Verification items for this drawing (mm, ordinates from the low corner). Round coordinates to 2 decimals unless told otherwise and drop trailing zeros. Loops run counter-clockwise (first coordinate to the right, second up) from the corner with the lowest first, then second, coordinate; pieces in that order, holes last. Notation, with made-up numbers: (28, 67) -> (65, 67) arc R24 cw to (65, 84) -> close; hole circle Ø1 at (77, 22). An arc over 180 degrees is marked (long way). Use a Markdown table: item, result. Add a question column.
Q1. Material ranges on L1, parallel to Y at x = 23.76, z = 2.7; L2, parallel to X at y = 31.5, z = 0.4; L3, parallel to Y at x = 24.5, z = 2.3, recorded low to high.
Q2. Sectioned sample at D-D, the plane x = 8. Enter the section's corners in (y, z).
Q3. Sectioned sample at A-A, the plane x = 23.76. Enter the section's corners in (y, z), then the cut area to 3 significant figures.
Q4. Sectioned sample at B-B, the plane y = 32.5. Enter the section's corners in (x, z).
Q5. Sectioned sample at C-C, the plane z = 2.25. Enter the section's corners in (x, y) (1 decimal).
Q6. Gauge pin test, flat ends, axial feed: P1, Ø1, axis at y = 57.5, z = 4, coming from the -X side (1 decimal); P2, Ø9, axis at x = 23.76, y = 32.5, coming from the +Z side. Record the tip position at first contact, or that the pin passes through.
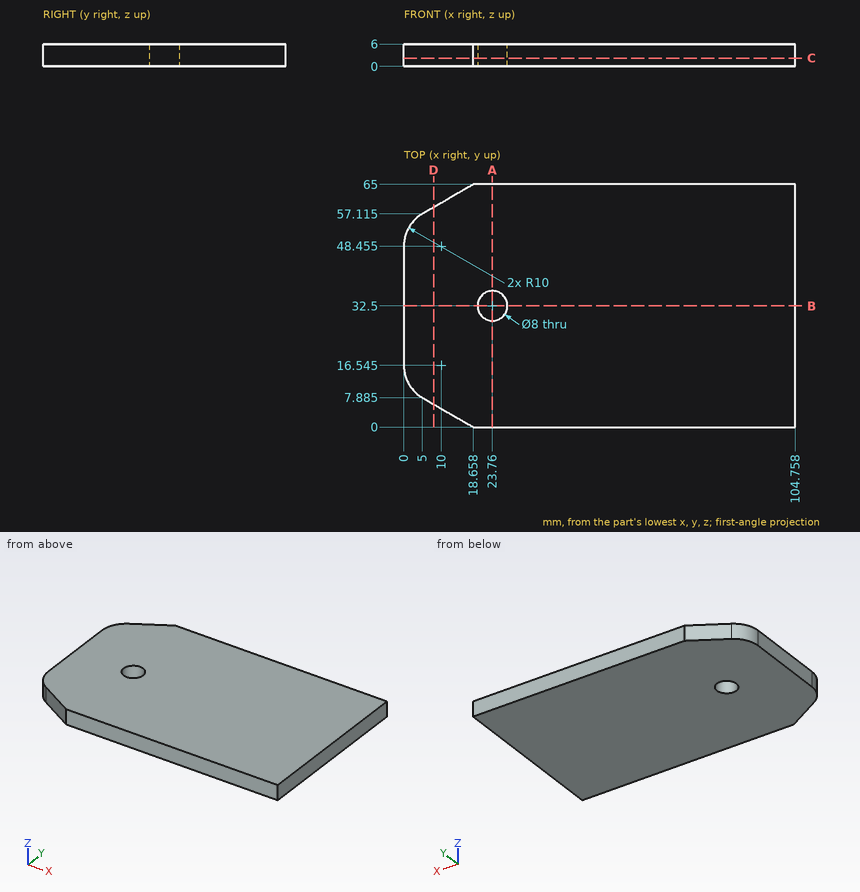
Values:
| question | item | result |
|---|---|---|
| 1 | L1 | 0 to 28.5, 36.5 to 65 |
| 1 | L2 | 0 to 19.89, 27.63 to 104.76 |
| 1 | L3 | 0 to 28.57, 36.43 to 65 |
| 2 | outline | (6.15, 0) -> (58.85, 0) -> (58.85, 6) -> (6.15, 6) -> close |
| 3 | outline | (0, 0) -> (28.5, 0) -> (28.5, 6) -> (0, 6) -> close; (36.5, 0) -> (65, 0) -> (65, 6) -> (36.5, 6) -> close |
| 3 | area | 342 mm^2 |
| 4 | outline | (0, 0) -> (19.76, 0) -> (19.76, 6) -> (0, 6) -> close; (27.76, 0) -> (104.76, 0) -> (104.76, 6) -> (27.76, 6) -> close |
| 5 | outline | (0, 16.5) arc R10 ccw to (5, 7.9) -> (18.7, 0) -> (104.8, 0) -> (104.8, 65) -> (18.7, 65) -> (5, 57.1) arc R10 ccw to (0, 48.5) -> close; hole circle Ø8 at (23.8, 32.5) |
| 6 | P1 | x = 4.8 |
| 6 | P2 | z = 6 |
